```python
from build123d import *

# Parameters (mm, degrees)
BOSS_EXTRUDE1_DEPTH      = 12
CUT_EXTRUDE1_DEPTH       = 2
SKETCH3_W                = 16.6
SKETCH3_H                = 15
BOSS_EXTRUDE2_DEPTH      = 5.2
SKETCH5_R                = 1.6
CUT_EXTRUDE2_DEPTH       = 5
SKETCH6_W                = 10
SKETCH6_H                = 4
BOSS_EXTRUDE4_DEPTH      = 8
CUT_EXTRUDE4_DEPTH       = 7
SKETCH8_R                = 2.65
CUT_EXTRUDE5_DEPTH       = 7
SKETCH10_R               = 2.65
CUT_EXTRUDE6_DEPTH       = 7
BOSS_EXTRUDE6_DEPTH      = 2
BOSS_EXTRUDE6_DEPTH_BACK = 7
SKETCH11_W               = 7
SKETCH11_H               = 3
CHAMFER2_SIZE            = 2


with BuildPart() as part:
    # Sketch1 → Boss-Extrude1 (new body)
    with BuildSketch(Plane(origin=(0, 0, 0), x_dir=(1, 0, 0), z_dir=(0, 1, 0))):
        with BuildLine():
            Line((-23.25, -5), (-5.749755012, -5))
            Line((-5.749755012, -5), (-5.749755012, 0))
            add(Edge.make_bspline(
                [(-3.25, 5), (-5.749755012, 5), (-5.749755012, 0)],
                knots=[0, 0, 0, 1.570796327, 1.570796327, 1.570796327], degree=2, weights=[1, 0.707106781, 1]))
            Line((-3.25, 5), (3.25, 5))
            add(Edge.make_bspline(
                [(5.748694825, 0), (5.748694825, 5), (3.25, 5)],
                knots=[4.71238898, 4.71238898, 4.71238898, 6.283185307, 6.283185307, 6.283185307], degree=2, weights=[1, 0.707106781, 1]))
            Line((5.748694825, 0), (5.748694825, -5))
            Line((5.748694825, -5), (23.25, -5))
            Line((23.25, -5), (23.25, -3))
            Line((23.25, -3), (23.25, -1))
            Line((23.25, -1), (9.3, -1))
            ThreePointArc((9.3, -1), (8.592893219, -0.707106781), (8.3, 0))
            Line((8.3, 0), (8.3, 6.6))
            Line((8.3, 6.6), (-8.3, 6.6))
            Line((-8.3, 6.6), (-8.3, 0))
            ThreePointArc((-8.3, 0), (-8.592893219, -0.707106781), (-9.3, -1))
            Line((-9.3, -1), (-23.25, -1))
            Line((-23.25, -1), (-23.25, -5))
        make_face()
    extrude(amount=BOSS_EXTRUDE1_DEPTH)

    # Sketch2 → Cut-Extrude1 (cut)
    with BuildSketch(Plane(origin=(0, 0, 1), x_dir=(-1, 0, 0), z_dir=(0, 0, -1))):
        Polygon((20.147177825, 6), (18.213054423, 9.35), (14.344807619, 9.35), (12.410684218, 6), (14.344807619, 2.65), (18.213054423, 2.65), align=None)
        Polygon((-12.542169585, 6), (-14.476292987, 9.35), (-18.34453979, 9.35), (-20.278663192, 6), (-18.34453979, 2.65), (-14.476292987, 2.65), align=None)
    extrude(amount=-CUT_EXTRUDE1_DEPTH, mode=Mode.SUBTRACT)

    # Sketch3 → Boss-Extrude2 (add)
    with BuildSketch(Plane(origin=(0, 12, 0), x_dir=(1, 0, 0), z_dir=(0, 1, 0))):
        with Locations((0, 14.1)):
            Rectangle(SKETCH3_W, SKETCH3_H)
    extrude(amount=-BOSS_EXTRUDE2_DEPTH)

    # Sketch5 → Cut-Extrude2 (cut)
    with BuildSketch(Plane(origin=(0, 0, 1), x_dir=(-1, 0, 0), z_dir=(0, 0, -1))):
        with Locations((-16.410416388, 6)):
            Circle(SKETCH5_R)
        with Locations((16.278931021, 6)):
            Circle(SKETCH5_R)
    extrude(amount=-CUT_EXTRUDE2_DEPTH, mode=Mode.SUBTRACT)

    # Sketch6 → Boss-Extrude4 (add)
    with BuildSketch(Plane(origin=(0, 12, 0), x_dir=(1, 0, 0), z_dir=(0, 1, 0))):
        with Locations((11.448694825, -3)):
            Rectangle(SKETCH6_W, SKETCH6_H)
    extrude(amount=BOSS_EXTRUDE4_DEPTH)

    # Sketch7 → Cut-Extrude4 (cut)
    with BuildSketch(Plane(origin=(0, 0, 1), x_dir=(-1, 0, 0), z_dir=(0, 0, -1))):
        with BuildLine():
            ThreePointArc((-6.448694825, 16), (-6.567716372, 16.785269427), (-6.914089597, 17.5))
            Line((-6.914089597, 17.5), (-7.999397269, 17.5))
            Line((-7.999397269, 17.5), (-7.999397269, 14.5))
            Line((-7.999397269, 14.5), (-6.914089597, 14.5))
            ThreePointArc((-6.914089597, 14.5), (-6.567716372, 15.214730573), (-6.448694825, 16))
        make_face()
        with BuildLine():
            Line((-7.999397269, 17.5), (-6.914089597, 17.5))
            ThreePointArc((-6.914089597, 17.5), (-11.748694825, 16), (-6.914089597, 14.5))
            Line((-6.914089597, 14.5), (-7.999397269, 14.5))
            Line((-7.999397269, 14.5), (-7.999397269, 17.5))
        make_face()
        with BuildLine():
            Line((-6.448694825, 14.5), (-6.448694825, 16))
            ThreePointArc((-6.448694825, 16), (-6.567716372, 15.214730573), (-6.914089597, 14.5))
            Line((-6.914089597, 14.5), (-6.448694825, 14.5))
        make_face()
        with BuildLine():
            Line((-6.448694825, 16), (-6.448694825, 17.5))
            Line((-6.448694825, 17.5), (-6.914089597, 17.5))
            ThreePointArc((-6.914089597, 17.5), (-6.567716372, 16.785269427), (-6.448694825, 16))
        make_face()
    extrude(amount=-CUT_EXTRUDE4_DEPTH, mode=Mode.SUBTRACT)

    # Sketch8 → Cut-Extrude5 (cut, along a direction that is not the sketch's normal)
    with BuildSketch(Plane(origin=(0, 12, 0), x_dir=(1, 0, 0), z_dir=(0, 1, 0))):
        with Locations((-4, 9.6)):
            Circle(SKETCH8_R)
    extrude(amount=-CUT_EXTRUDE5_DEPTH, dir=(0.2588190451025147, 0.96592582628907, -1.457918124587514e-13), mode=Mode.SUBTRACT)

    # Sketch10 → Cut-Extrude6 (cut, along a direction that is not the sketch's normal)
    with BuildSketch(Plane(origin=(0, 12, 0), x_dir=(1, 0, 0), z_dir=(0, 1, 0))):
        with Locations((4, 9.6)):
            Circle(SKETCH10_R)
    extrude(amount=-CUT_EXTRUDE6_DEPTH, dir=(-0.25881904510251447, 0.96592582628907, 0), mode=Mode.SUBTRACT)

    # Sketch11 → Boss-Extrude6 (add, two sides: drawn at the far end of the back side and taken through both)
    with BuildSketch(Plane(origin=(0, 12, 0), x_dir=(1, 0, 0), z_dir=(0, 1, 0)).offset(-BOSS_EXTRUDE6_DEPTH_BACK)):
        with Locations((4.8, 14.5)):
            Rectangle(SKETCH11_W, SKETCH11_H)
    extrude(amount=BOSS_EXTRUDE6_DEPTH + BOSS_EXTRUDE6_DEPTH_BACK)

    # Chamfer2
    # the kernel refuses this chamfer: 2 mm, written as the material it takes off along each edge
    with BuildSketch(Plane(origin=(13.443365976, 5, -13), x_dir=(0, 0.9996219169112968, 0.027495876610586487), z_dir=(-1, 0, 0))) as chamfer2_piece_1_section:
        Polygon((CHAMFER2_SIZE * 0.999621916911, CHAMFER2_SIZE * 0.0274958766106), (-CHAMFER2_SIZE * 0.0274958766106, CHAMFER2_SIZE * 0.999621916911), (0, 0), align=None)
    chamfer2_piece_1 = extrude(amount=17.286731952, mode=Mode.PRIVATE)
    chamfer2_piece_1 = split(chamfer2_piece_1, bisect_by=Plane(origin=(4.8, 6.8, -13.671801494), z_dir=(0, -1, 0)), keep=Keep.TOP, mode=Mode.PRIVATE)
    add(chamfer2_piece_1, mode=Mode.SUBTRACT)
    with BuildSketch(Plane(origin=(13.443365976, 14, -13), x_dir=(0, -0.9996219169112968, 0.027495876610586487), z_dir=(-1, 0, 0))) as chamfer2_piece_2_section:
        Polygon((CHAMFER2_SIZE * 0.999621916911, -CHAMFER2_SIZE * 0.0274958766106), (-CHAMFER2_SIZE * 0.0274958766106, -CHAMFER2_SIZE * 0.999621916911), (0, 0), align=None)
    chamfer2_piece_2 = extrude(amount=17.286731952, mode=Mode.PRIVATE)
    chamfer2_piece_2 = split(chamfer2_piece_2, bisect_by=Plane(origin=(4.8, 12, -13.660808309), z_dir=(0, 1, 0)), keep=Keep.TOP, mode=Mode.PRIVATE)
    add(chamfer2_piece_2, mode=Mode.SUBTRACT)


solid = part.part
```
Read the model definition and answer for the solid it produces. Units are mm, in the model's axes. A direction names the side the tool comes from. Round coordinates to 2 decimals unless told otherwise and drop trailing zeros. Write each loop counter-clockwise with the first axis right and the second up, starting at its lowest first coordinate (ties: lowest second). Pieces come first, ordered by that corner, then holes. Notation, with made-up numbers: (38.5, -5.75) -> (73.5, -5.75) arc R13 cw to (73.5, 2.25) -> close; hole circle Ø6 at (54.25, 84.25). An arc over 180 degrees is marked (long way). Answer in a Markdown table with one row per item. Add a question column.
1) Find section B-B, the plane z = -15.5. Determine the outline of the cut face in (x, y).
2) Find section D-D, the plane x = 17. Determine the outline of the cut face in (y, z), and give its area (3 significant figures).
3) Given P1, Ø0.5, axis at y = 5.5, z = -14.5, coming from the -X side; P2, Ø2, axis at x = 0, y = 15.5, coming from the +Z side; P3, Ø5, axis at x = 16.41, y = 6, coming from the -Z side; P4, Ø4, axis at x = -16.28, y = 6, coming from the +Z side, each flat-ended and moving along its own axis, determine where each tip first touches the part or whether it passes through.
4) Which of the six approach directions +Z, -Z, +X, -X, +Y, -Y give full straight-line access (tool end or side, diameter ignored) to faces 4 (the face through (13.496, 7.652, 1.986)), 5 (the face through (5, 13, -14)), 6 (the face through (4.8, 5, -15.5)), 7 (the face through (8.3, 8, -8))?
5) Find section A-A, the plane x = -15.5. Determine the outline of the cut face in (y, z).
6) Consider line 1 (X direction, y = 5.25, z = -15); line 2 (Y direction, x = 9, z = 2.25); line 3 (Z direction, x = 12, y = 12.75). Determine where each line is inside the solid, lowest interval first.
7) Find section C-C, the plane y = 16. Determine the outline of the cut face in (x, z).
8) Determine the mould class of faces 1 (the face through (0, 6, -5)), 2 (the face through (-8.585, 5.916, 0.699)), 3 (the face through (11, 20, 3)) for opening direction X: pulls with the +X half, pulls with the -X half, needs draft (parallel to the pull), parting line crosses it, or undercut.
Findings below:
| question | item | result |
|---|---|---|
| 1 | outline | (-8.3, 6.8) -> (1.3, 6.8) -> (1.3, 5) -> (8.3, 5) -> (8.3, 14) -> (1.3, 14) -> (1.3, 12) -> (-8.3, 12) -> close |
| 2 | outline | (0, 1) -> (2.65, 1) -> (2.65, 3) -> (4.51, 3) -> (4.51, 5) -> (0, 5) -> close; (7.49, 3) -> (9.35, 3) -> (9.35, 1) -> (12, 1) -> (12, 5) -> (7.49, 5) -> close |
| 2 | area | 28.7 mm² |
| 3 | P1 | x = 1.3 |
| 3 | P2 | through |
| 3 | P3 | z = 3 |
| 3 | P4 | z = 5 |
| 4 | face 4 | -Z |
| 4 | face 5 | +X, -X, +Y |
| 4 | face 6 | -Z, +X, -X, -Y |
| 4 | face 7 | -Z, +X, +Y, -Y |
| 5 | outline | (0, 1) -> (2.65, 1) -> (2.65, 3) -> (4.6, 3) -> (4.6, 5) -> (0, 5) -> close; (7.4, 3) -> (9.35, 3) -> (9.35, 1) -> (12, 1) -> (12, 5) -> (7.4, 5) -> close |
| 6 | line 1 | 1.3 to 8.3 |
| 6 | line 2 | 0 to 13.35, 18.65 to 20 |
| 6 | line 3 | 1 to 5 |
| 7 | outline | (11.75, 1) -> (16.45, 1) -> (16.45, 5) -> (11.75, 5) -> close |
| 8 | face 1 | undercut |
| 8 | face 2 | pulls with the -X half |
| 8 | face 3 | needs draft |
